Work out the finished part from the listing and answer in its coordinate system (mm). A direction names the side the tool comes from. Give positions to 0.01 mm unless a question says otherwise; leave off trailing zeros. Loops run counter-clockwise (first coordinate to the right, second up) from the corner with the lowest first, then second, coordinate; pieces in that order, holes last. Notation, with made-up numbers: M 19.25,55.25 L 54.25,55.25 A17 cw 54.25,68.25 Z; hole C -13.5,61.5 d11. An arc over 180 degrees is marked long. Use a Markdown table: item, result.
```python
from build123d import *

# Parameters (mm, degrees)
CUT_EXTRUDE_1_DEPTH = 1.2
CUT_EXTRUDE_2_DEPTH = 2.7


with BuildPart() as part:
    # Sketch 1 → Revolve 1 (revolve)
    with BuildSketch(Plane.XY, mode=Mode.PRIVATE) as revolve_1_sk:
        with BuildLine():
            Line((0, 0), (0, 2.5))
            Line((0, 2.5), (0.5, 3))
            Line((0.5, 3), (34.5, 3))
            ThreePointArc((34.5, 3), (34.853553391, 3.146446609), (35, 3.5))
            Line((35, 3.5), (35, 9.5))
            Line((35, 9.5), (35.5, 10))
            Line((35.5, 10), (50.5, 10))
            ThreePointArc((50.5, 10), (50.853553391, 10.146446609), (51, 10.5))
            Line((51, 10.5), (51, 14.5))
            Line((51, 14.5), (51.5, 15))
            Line((51.5, 15), (76.5, 15))
            Line((76.5, 15), (77, 14.5))
            Line((77, 14.5), (77, 0))
            Line((77, 0), (0, 0))
        make_face()
    revolve(revolve_1_sk.sketch.rotate(Axis((0, 0, 0), (1, 0, 0)), 90), axis=Axis((0, 0, 0), (1, 0, 0)))

    # Sketch 3 → Cut-Extrude 1 (cut)
    with BuildSketch(Plane.XY.offset(10)):
        with BuildLine():
            Line((39, 3), (47, 3))
            ThreePointArc((47, 3), (50, 0), (47, -3))
            Line((47, -3), (39, -3))
            ThreePointArc((39, -3), (36, 0), (39, 3))
        make_face()
    extrude(amount=-CUT_EXTRUDE_1_DEPTH, mode=Mode.SUBTRACT)

    # Sketch 4 → Cut-Extrude 2 (cut)
    with BuildSketch(Plane.XY.offset(15)):
        with BuildLine():
            Line((58, 5), (70, 5))
            ThreePointArc((70, 5), (75, 0), (70, -5))
            Line((70, -5), (58, -5))
            ThreePointArc((58, -5), (53, 0), (58, 5))
        make_face()
    extrude(amount=-CUT_EXTRUDE_2_DEPTH, mode=Mode.SUBTRACT)


solid = part.part
```
(1) Which of the six approach directions +Z, -Z, +X, -X, +Y, -Y give full straight-line access (tool end or side, diameter ignored) to faces 1 (the flat face through (0, 0, 0)), 2 (the cylindrical face through (50, 0, 9)), 3 (the flat face through (35, 0, -4))?
Entries:
| item | result |
|---|---|
| face 1 | +Z, -Z, -X, +Y, -Y |
| face 2 | +Z |
| face 3 | -X |
(2) A cutting plane is placed at A-A (z = 0). Write down the section's boundary in (x, y).
Entries:
| item | result |
|---|---|
| outline | M 0,-2.5 L 0.5,-3 L 34.5,-3 A0.5 cw 35,-3.5 L 35,-9.5 L 35.5,-10 L 50.5,-10 A0.5 cw 51,-10.5 L 51,-14.5 L 51.5,-15 L 76.5,-15 L 77,-14.5 L 77,14.5 L 76.5,15 L 51.5,15 L 51,14.5 L 51,10.5 A0.5 cw 50.5,10 L 35.5,10 L 35,9.5 L 35,3.5 A0.5 cw 34.5,3 L 0.5,3 L 0,2.5 Z |
(3) Given P1, Ø12, axis at x = 8.5, y = 6.5, coming from the +Z side; P2, Ø10, axis at y = -7, z = -3.5, coming from the -X side; P3, Ø1.5, axis at x = 62, z = 13, coming from the -Y side, each flat-ended and moving along its own axis, determine where each tip first touches the part or whether it passes through.
Entries:
| item | result |
|---|---|
| P1 | stops at z = 2.96 |
| P2 | stops at x = 0.33 |
| P3 | stops at y = -8.66 |
(4) A cutting plane is placed at D-D (x = 27). Write down the section's boundary in (y, z).
Entries:
| item | result |
|---|---|
| outline | C 0,0 d6 |
(5) The mould has two halves that part along X. Classify faces 4 (the flat face through (43, 0, 8.8)), 5 (the flat face through (77, 0, 0)), 6 (the cylindrical face through (36, 0, 9)), 7 (the cylindrical face through (17.74, -0.9, 2.86)): released by +X, released by -X, zero draft, split by the parting line, or undercut.
Entries:
| item | result |
|---|---|
| face 4 | undercut |
| face 5 | released by +X |
| face 6 | undercut |
| face 7 | zero draft |
(6) A cutting plane is placed at C-C (x = 65). Write down the section's boundary in (y, z).
Entries:
| item | result |
|---|---|
| outline | M -5,12.3 L -5,14.14 A15 ccw long 5,14.14 L 5,12.3 Z |
(7) Consider probe 1 along X at (y, z) = (4.5, -1.5); probe 2 along X at (y, z) = (10, -7); probe 3 along Z at (x, y) = (74, -8.5). Determine where each line is inside the solid, lowest interval first. Write a range as [from, to].
Entries:
| item | result |
|---|---|
| probe 1 | x = [35, 77] |
| probe 2 | x = [51, 77] |
| probe 3 | z = [-12.36, 12.36] |
